from build123d import *

# Parameters (mm, degrees)
F0_R      = 359.41
F1_DEPTH  = 300
F2_R      = 504.3357911894
F2_R_2    = 155
F3_DEPTH  = 260
F4_R      = 50.8
F5_R      = 125
F6_DEPTH  = 708.66
F7_R      = 9.525
F8_DEPTH  = 109.22
F10_DEPTH = 340.868


with BuildPart() as f1:
    # F0 (on Front) → F1 (new body)
    with BuildSketch(Plane.XZ):
        Circle(F0_R)
    extrude(amount=F1_DEPTH)

    # F2 (on face) → F3 (cut)
    with BuildSketch(Plane.XZ.offset(300)):
        Circle(F2_R)
        Circle(F2_R_2, mode=Mode.SUBTRACT)
    extrude(amount=-F3_DEPTH, mode=Mode.SUBTRACT)

    # F4
    f4_edges = [f1.edges().sort_by_distance(p)[0] for p in [
        (-155, -40, 0),
    ]]
    fillet(f4_edges, radius=F4_R)

    # F5 (on face) → F6 (cut)
    with BuildSketch(Plane.XZ.offset(300)):
        Circle(F5_R)
    extrude(amount=-F6_DEPTH, mode=Mode.SUBTRACT)

    # F7 (on face) → F8 (cut)
    with BuildSketch(Plane.XZ.offset(40)):
        with Locations((0, 342.9)):
            Circle(F7_R)
        with Locations((-66.8964714193, 336.3112726503)):
            Circle(F7_R)
        with Locations((-131.222148958, 316.7982916981)):
            Circle(F7_R)
        with Locations((-190.5050329024, 285.1109300585)):
            Circle(F7_R)
        with Locations((-242.4669152689, 242.4669152689)):
            Circle(F7_R)
        with Locations((-285.1109300585, 190.5050329024)):
            Circle(F7_R)
        with Locations((-316.7982916981, 131.222148958)):
            Circle(F7_R)
        with Locations((-336.3112726503, 66.8964714193)):
            Circle(F7_R)
        with Locations((-342.9, 0)):
            Circle(F7_R)
        with Locations((-336.3112726503, -66.8964714193)):
            Circle(F7_R)
        with Locations((-316.7982916981, -131.222148958)):
            Circle(F7_R)
        with Locations((-285.1109300585, -190.5050329024)):
            Circle(F7_R)
        with Locations((-242.4669152689, -242.4669152689)):
            Circle(F7_R)
        with Locations((-190.5050329024, -285.1109300585)):
            Circle(F7_R)
        with Locations((-131.222148958, -316.7982916981)):
            Circle(F7_R)
        with Locations((-66.8964714193, -336.3112726503)):
            Circle(F7_R)
        with Locations((0, -342.9)):
            Circle(F7_R)
        with Locations((66.8964714193, -336.3112726503)):
            Circle(F7_R)
        with Locations((131.222148958, -316.7982916981)):
            Circle(F7_R)
        with Locations((190.5050329024, -285.1109300585)):
            Circle(F7_R)
        with Locations((242.4669152689, -242.4669152689)):
            Circle(F7_R)
        with Locations((285.1109300585, -190.5050329024)):
            Circle(F7_R)
        with Locations((316.7982916981, -131.222148958)):
            Circle(F7_R)
        with Locations((336.3112726503, -66.8964714193)):
            Circle(F7_R)
        with Locations((342.9, 0)):
            Circle(F7_R)
        with Locations((336.3112726503, 66.8964714193)):
            Circle(F7_R)
        with Locations((316.7982916981, 131.222148958)):
            Circle(F7_R)
        with Locations((285.1109300585, 190.5050329024)):
            Circle(F7_R)
        with Locations((242.4669152689, 242.4669152689)):
            Circle(F7_R)
        with Locations((190.5050329024, 285.1109300585)):
            Circle(F7_R)
        with Locations((131.222148958, 316.7982916981)):
            Circle(F7_R)
        with Locations((66.8964714193, 336.3112726503)):
            Circle(F7_R)
    extrude(amount=-F8_DEPTH, mode=Mode.SUBTRACT)

    # F9 (on face) → F10 (cut)
    with BuildSketch(Plane.XZ.offset(300)):
        with BuildLine():
            Line((0, 125), (0, 0))
            Line((0, 0), (25.4, 0))
            Line((25.4, 0), (25.4, 122.3921566114))
            ThreePointArc((25.4, 122.3921566114), (12.766761993, 124.3463300151), (0, 125))
        make_face()
        with BuildLine():
            ThreePointArc((-25.4, 122.3921566114), (-12.766761993, 124.3463300151), (0, 125))
            Line((0, 125), (0, 139.0471624903))
            Line((0, 139.0471624903), (-25.4, 139.0471624903))
            Line((-25.4, 139.0471624903), (-25.4, 122.3921566114))
        make_face()
        with BuildLine():
            Line((-25.4, 0), (0, 0))
            Line((0, 0), (0, 125))
            ThreePointArc((0, 125), (-12.766761993, 124.3463300151), (-25.4, 122.3921566114))
            Line((-25.4, 122.3921566114), (-25.4, 0))
        make_face()
        with BuildLine():
            Line((0, 139.0471624903), (0, 125))
            ThreePointArc((0, 125), (12.766761993, 124.3463300151), (25.4, 122.3921566114))
            Line((25.4, 122.3921566114), (25.4, 139.0471624903))
            Line((25.4, 139.0471624903), (0, 139.0471624903))
        make_face()
    extrude(amount=-F10_DEPTH, mode=Mode.SUBTRACT)


solid = f1.part
Read the model definition and answer for the solid it produces. Units are mm, in the model's axes. Round coordinates to 2 decimals unless told otherwise and drop trailing zeros. Order: outer loops, then holes, each group sorted by start corner. A loop starts at its lowest first (then second) coordinate and runs counter-clockwise, first axis right, second up.
1) The part is cut by section D-D on x = -266. Write down the section's boundary in (y, z), plus the area to 3 significant figures.
2) The part is cut by section B-B on y = -215. Write down the section's boundary in (x, z).
3) The mould has two halves that part along Z. Classify faces 1 (the face through (-68.136, -20.28, 345.755)), 2 (the face through (-77.913, -19.72, -350.863)), 3 (the face through (155, -40, -155)): released by +Z, released by -Z, zero draft, split by the parting line, or undercut.
4) The part is cut by section C-C on y = -64. Write down the section's boundary in (x, z).
5) Flat-ended cylindrical pins translate along their axes: pin 1 (1 mm diameter, centred on y = -112, z = -138.5, fed in from -X); pin 2 (13.5 mm diameter, centred on y = -111, z = 128, fed in from -X); pin 3 (22 mm diameter, centred on x = 131.22, z = 316.8, fed in from -Y). Find the tip coordinate at first contact, or state that the pin passes through.
6) The part is cut by section A-A on x = 0. Write down the section's boundary in (y, z) (3 decimals).
7) Straight lines are drawn through the part: L1, parallel to Y at x = -256.5, z = -161; L2, parallel to Z at x = -10, y = -171; L3, parallel to X at y = -194, z = 75. For each, find the intervals that lie inside material, in ascending order.
Resolved:
1. outline: (-40, -241.7) - (0, -241.7) - (0, 241.7) - (-40, 241.7) - close
1. area: 19,300 mm2
2. outline: circle Ø310 at (0, 0); hole (-25.4, 122.39) arc R125 ccw (long way) to (25.4, 122.39) - (25.4, 139.05) - (-25.4, 139.05) - close
3. face 1: undercut
3. face 2: split by the parting line
3. face 3: zero draft
4. outline: circle Ø325.29 at (0, 0); hole (-25.4, 122.39) arc R125 ccw (long way) to (25.4, 122.39) - (25.4, 139.05) - (-25.4, 139.05) - close
5. pin 1: stops at x = -70.58
5. pin 2: stops at x = -96.56
5. pin 3: stops at y = -40
6. outline: (-300, -155) - (-90.8, -155) arc R50.8 cw to (-40, -205.8) - (-40, -333.375) - (0, -333.375) - (0, -125) - (-300, -125) - close; (-300, 139.047) - (0, 139.047) - (0, 333.375) - (-40, 333.375) - (-40, 205.8) arc R50.8 cw to (-90.8, 155) - (-300, 155) - close; (-40, -359.41) - (0, -359.41) - (0, -352.425) - (-40, -352.425) - close; (-40, 352.425) - (0, 352.425) - (0, 359.41) - (-40, 359.41) - close
7. L1: y = -40 to 0
7. L2: z = -154.68 to -124.6, 139.05 to 154.68
7. L3: x = -135.65 to -100, 100 to 135.65
